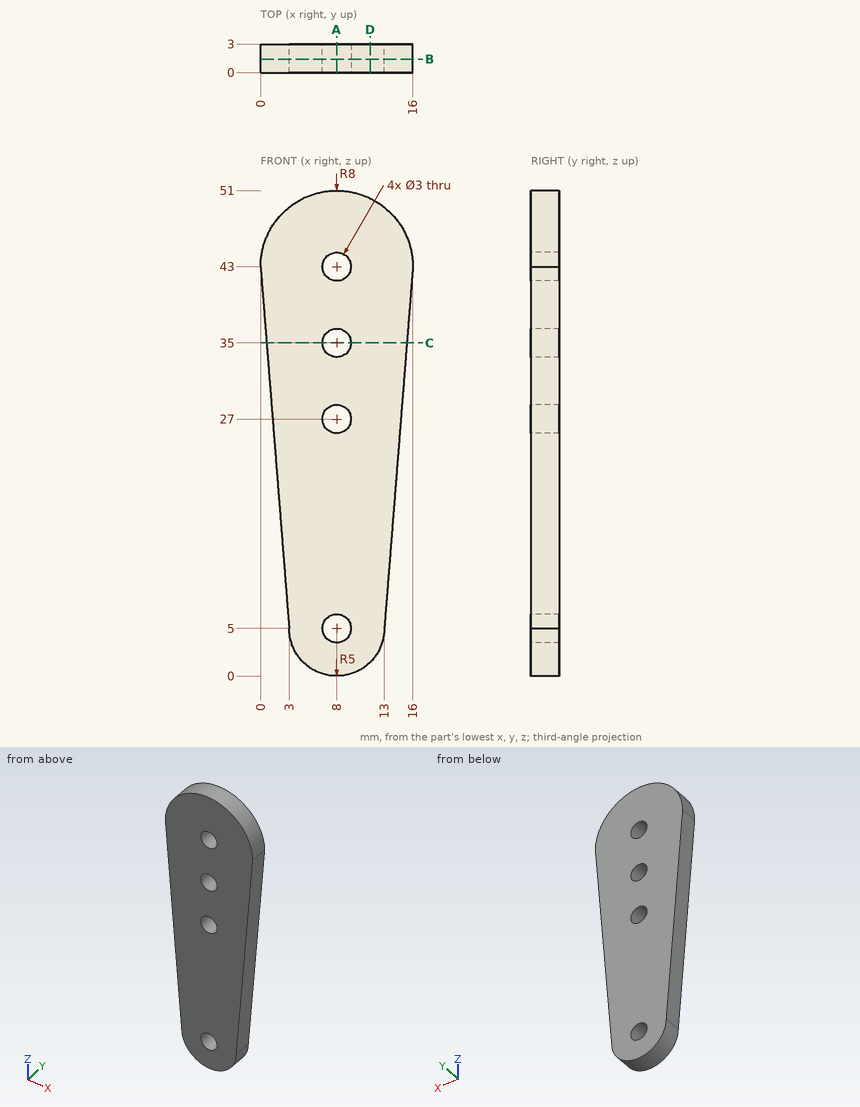
Source: three-view drawing plus pictorial views. Frame: mm from the lowest corner of the part. Coordinates: 2 decimals unless noted, no trailing zeros. Order: outer loops, then holes, each group sorted by start corner. A loop starts at its lowest first (then second) coordinate and runs counter-clockwise, first axis right, second up.
Item 1: Cut plane B-B (y = 1.4). Return loops of the section in (x, z).
Output values:
outline: (0, 43) - (3, 5) arc R5 ccw to (13, 5) - (16, 43) arc R8 ccw to start; hole circle Ø3 at (8, 5); hole circle Ø3 at (8, 27); hole circle Ø3 at (8, 35); hole circle Ø3 at (8, 43)
Item 2: Cut plane D-D (x = 11.5). Return loops of the section in (y, z), plus the area to 3 significant figures.
Output values:
outline: (0, 1.43) - (3, 1.43) - (3, 50.19) - (0, 50.19) - close
area: 146 mm2
Item 3: Cut plane A-A (x = 8). Return loops of the section in (y, z).
Output values:
outline: (0, 0) - (3, 0) - (3, 3.5) - (0, 3.5) - close; (0, 6.5) - (3, 6.5) - (3, 25.5) - (0, 25.5) - close; (0, 28.5) - (3, 28.5) - (3, 33.5) - (0, 33.5) - close; (0, 36.5) - (3, 36.5) - (3, 41.5) - (0, 41.5) - close; (0, 44.5) - (3, 44.5) - (3, 51) - (0, 51) - close
Item 4: Material intervals for line 1 (Z direction, x = 8, y = 1.9); line 2 (Z direction, x = 9.25, y = 2.6) (1 decimal); line 3 (X direction, y = 1.9, z = 40), sorted ascending.
Output values:
line 1: z = 0 to 3.5, 6.5 to 25.5, 28.5 to 33.5, 36.5 to 41.5, 44.5 to 51
line 2: z = 0.2 to 4.2, 5.8 to 26.2, 27.8 to 34.2, 35.8 to 42.2, 43.8 to 50.9
line 3: x = 0.24 to 15.76
Item 5: First-contact query: P1, Ø5, axis at x = 8, z = 27, coming from the +Y side; P2, Ø2.5, axis at x = 8, z = 5, coming from the +Y side; P3, Ø1, axis at y = 1, z = 27.5, coming from the +X side. Flat tips, straight axial feed; report the tip coordinate or a pass-through.
Output values:
P1: stops at y = 3
P2: passes through
P3: stops at x = 14.82
Item 6: Cut plane C-C (z = 35). Return loops of the section in (x, y).
Output values:
outline: (0.63, 0) - (6.5, 0) - (6.5, 3) - (0.63, 3) - close; (9.5, 0) - (15.37, 0) - (15.37, 3) - (9.5, 3) - close
